Autodesk Inventor part; units mm, degrees
ref_plane "YZ Plane" through (0, 0, 0) normal (1, 0, 0) x (0, 1, 0)
ref_plane "XZ Plane" through (0, 0, 0) normal (0, 1, 0) x (-1, 0, 0)
ref_plane "XY Plane" through (0, 0, 0) normal (0, 0, 1) x (1, 0, 0)
sketch "Sketch1" plane through (0, 0, 0) normal (0, 0, 1) x (1, 0, 0)
  line L0 (4.25, 0) -> (4.25, 4.5)
  line L1 (4.25, 4.5) -> (0, 4.5)
  line L2 (4.25, 0) -> (1.75, 0)
  line L3 (1.75, 0) -> (1.75, -8)
  line L4 (1.75, -8) -> (2.5, -8)
  line L5 (2.5, -8) -> (2.5, -14)
  line L6 (2.5, -14) -> (0, -14)
  line L7 (0, 4.5) -> (0, -14)
  point P0 (0, 0)
  dimension "d0" = 8.5
  dimension "d2" = 3.5
  dimension "d3" = 5
  dimension "d4" = 4.5
  dimension "d5" = 6
  dimension "d6" = 14
revolve "Вращение1" add sketch "Sketch1" angle 360 about axis through (0, 4.5, 0) along (0, -1, 0)
sketch "Sketch2" plane through (0, 4.5, 0) normal (0, 1, 0) x (1, 0, 0)
  circle A0 centre (0, 0) radius 4.25 construction
  circle A1 centre (0, 0) radius 1.25
  dimension "d31" = 2.5
extrude "Выдавливание1" cut sketch "Sketch2" against normal blind 1.5
chamfer "Фаска1" distance 0.9 angle 45 1 edges at (-4.25, 4.5, 0)
sketch "Sketch3" plane through (0, 0, 0) normal (0, 0, 1) x (1, 0, 0)
  line L0 (0, 0) -> (0, 4.5)
  line L1 (-2.3552, 0) -> (2.3552, 0) construction
  line L2 (-4.25, 4.5) -> (4.25, 4.5) construction
  line L3 (-0.6, 4.5) -> (0.6, 4.5)
  line L4 (0.6, 4.5) -> (0.6, 1.3)
  line L5 (0.6, 1.3) -> (-0.6, 1.3)
  line L6 (-0.6, 1.3) -> (-0.6, 4.5)
  dimension "d8" = 1.3
  dimension "d9" = 1.2
extrude "Выдавливание2" cut sketch "Sketch3" along normal through all both and the other way through all
fillet "Сопряжение1" radius 0.4 2 edges at (-1.75, 0, 0) (-1.75, -8, 0)
thread "Резьба1"
chamfer "Фаска2" distance 0.9 angle 45 1 edges at (-2.5, -14, 0)
equation "\"d31\" = d3_"
equation "\"d32\" = h3"
equation "\"d21\" = C1"
equation "\"d8\" = h2"
equation "\"d9\" = n"
equation "\"d12\" = R"
equation "\"d13\" = b"
equation "\"d15\" = C1"
equation "\"d0\" = D"
equation "\"d2\" = d1"
equation "\"d3\" = d_"
equation "\"d4\" = k1"
equation "\"d5\" = b"
equation "\"d6\" = l_"
equation "\"D\" = 8.5"
equation "\"d_\" = 5"
equation "\"l_\" = 14"
equation "\"b\" = 6"
equation "\"d1\" = 3.5"
equation "\"R\" = 0.4"
equation "\"C1\" = 0.9"
equation "\"h2\" = 1.3"
equation "\"n\" = 1.2"
equation "\"h3\" = 1.5"
equation "\"k1\" = 4.5"
equation "\"d3_\" = 2.5"
equation "\"G\" = l_ - b"
properties part number "Винт 3 M5-6gx14 ГОСТ 10336-80" material "Сталь, мягкая"
Here's how the part is built. I have some questions about the finished solid (model axes, mm). A direction names the side the tool comes from. Give positions to 0.01 mm unless a question says otherwise; leave off trailing zeros. Write each loop counter-clockwise with the first axis right and the second up, starting at its lowest first coordinate (ties: lowest second). Pieces come first, ordered by that corner, then holes. Notation, with made-up numbers: (56, -34) -> (108, -34) arc R26 ccw to (108, -3) -> close; hole circle Ø9 at (70, 12). An arc over 180 degrees is marked (long way). Write each question's results on one line, items separated by ' | '.
Item 1: Suppose I cut it at A-A on z = 0. Write out the boundary of the cut face in (x, y).
Output:
outline: (-4.25, 0) -> (-2.15, 0) arc R0.4 cw to (-1.75, -0.4) -> (-1.75, -7.6) arc R0.4 cw to (-2.15, -8) -> (-2.5, -8) -> (-2.5, -13.1) -> (-1.6, -14) -> (1.6, -14) -> (2.5, -13.1) -> (2.5, -8) -> (2.15, -8) arc R0.4 cw to (1.75, -7.6) -> (1.75, -0.4) arc R0.4 cw to (2.15, 0) -> (4.25, 0) -> (4.25, 3.6) -> (3.35, 4.5) -> (1.25, 4.5) -> (1.25, 3) -> (0.6, 3) -> (0.6, 1.3) -> (-0.6, 1.3) -> (-0.6, 3) -> (-1.25, 3) -> (-1.25, 4.5) -> (-3.35, 4.5) -> (-4.25, 3.6) -> close
Item 2: For pin 1 Ø1.5 at (x, y) = (0, -12) entering from -Z; pin 2 Ø4 at (y, z) = (-10, -2) entering from -X; pin 3 Ø1 at (x, z) = (0, 2) entering from +Y, each with a flat end and sliding along its axis, tell me the tip position at first contact or that it passes through.
Output:
pin 1: stops at z = -2.5 | pin 2: stops at x = -2.5 | pin 3: stops at y = 1.3
Item 3: If I drill on L1, parallel to Y at x = 0, z = 1.25; L2, parallel to Y at x = -1, z = 3; L3, parallel to Z at x = 0, y = -0.5, over which ranges is the centre line in solid material (lowest first)?
Output:
L1: y = -14 to 1.3 | L2: y = 0 to 4.5 | L3: z = -1.75 to 1.75
Item 4: Suppose I cut it at D-D on y = -3. Write out the boundary of the cut face in (x, z).
Output:
outline: circle Ø3.5 at (0, 0)
Item 5: We'd pull the mould along X, two halves only. Please class faces 5 (the face through (0, -14, 0)), 6 (the face through (-3.51, 4.34, 0.07)), 7 (the face through (0.6, 2.6, -0.1)): pulls with the +X half, pulls with the -X half, needs draft (parallel to the pull), parting line crosses it, or undercut.
Output:
face 5: needs draft | face 6: pulls with the -X half | face 7: undercut
Item 6: Suppose I cut it at C-C on x = 0. Write out the boundary of the cut face in (y, z), plus the area to 3 significant figures.
Output:
outline: (-14, -1.6) -> (-13.1, -2.5) -> (-8, -2.5) -> (-8, -2.15) arc R0.4 cw to (-7.6, -1.75) -> (-0.4, -1.75) arc R0.4 cw to (0, -2.15) -> (0, -4.25) -> (1.3, -4.25) -> (1.3, 4.25) -> (0, 4.25) -> (0, 2.15) arc R0.4 cw to (-0.4, 1.75) -> (-7.6, 1.75) arc R0.4 cw to (-8, 2.15) -> (-8, 2.5) -> (-13.1, 2.5) -> (-14, 1.6) -> close | area: 68.4 mm^2
Item 7: On a 3-axis mill with a long thin cutter (end or side, diameter ignored), from which of +Z, -Z, +X, -X, +Y, -Y can I reach the whole of each face in a straight line? I mean faces 1 (the face through (-1.25, 3.76, -0.02)), 2 (the face through (-0.54, -10.59, -2.44)), 3 (the face through (1.617, -4.05, -0.67)), 4 (the face through (-0.6, 2.5, -0.1)). Say none if no direction works.
Output:
face 1: +Y | face 2: -Y | face 3: none | face 4: +Z, -Z, +Y
Item 8: Suppose I cut it at B-B on y = 2.25. Write out the boundary of the cut face in (x, z), plus the area to 3 significant figures.
Output:
outline: (-0.6, -4.21) -> (-0.6, 4.21) arc R4.25 ccw to start; (0.6, -4.21) arc R4.25 ccw to (0.6, 4.21) -> close | area: 46.6 mm^2
